Read the model definition and answer for the solid it produces. Units are mm, in the model's axes. A direction names the side the tool comes from. Coordinates: 2 decimals unless noted, no trailing zeros. Write each loop counter-clockwise with the first axis right and the second up, starting at its lowest first coordinate (ties: lowest second). Pieces come first, ordered by that corner, then holes.
Item 1: Determine the mould class of faces 1 (the face through (100, -3, 3)), 2 (the face through (1, -133.919, 3)), 3 (the face through (-76, -81, 3)) for opening direction Y: released by +Y, released by -Y, zero draft, split by the parting line, or undercut.
Item 2: Section A-A (x = 18) is taken. Give the vertices of the cut face in (y, z).
Item 3: Section B-B (y = -28) is taken. Give the vertices of the cut face in (x, z), then the cut area to 3 significant figures.
Item 4: Straight lines are drawn through the part: probe 1 along Y at (x, z) = (-11.5, 5.75); probe 2 along X at (y, z) = (-106, 5); probe 3 along X at (y, z) = (-68, 1.25). For each, find the intervals that lie inside material, in ascending order.
Item 5: Section C-C (z = 5.25) is taken. State how many separate pieces and enclosed holes the cut face has, then the cut area to 3 significant figures.
Item 6: A tool of negligible diameter and unlimited length cuts with its end or side. For faces 4 (the face through (34.308, 33.056, 3.131)), 5 (the face through (1, -29, 0)), from which of +Z, -Z, +X, -X, +Y, -Y can it reach the whole face along a straight path? Write none if from no direction.
Item 7: Each of these flat-tipped pins is pushed along its axis until it touches: P1, Ø12, axis at x = 24, y = 68, coming from the -Z side; P2, Ø3.5, axis at x = -88.37, y = -112.21, coming from the -Z side. Where does it stop, or does it pass through?
from build123d import *

# Parameters (mm, degrees)
SKETCH1_W                   = 100
SKETCH1_H                   = 265.76692074
SKETCH1_R                   = 3
BOSS_EXTRUDE2_DEPTH         = 6.35
CUTOUT_FILLETS_R            = 5
CUTOUT_FILLETS_OF_MIRROR2_R = 5


with BuildPart() as part:
    # Sketch1 → Boss-Extrude2 (new body)
    with BuildSketch(Plane.XY):
        with Locations((50, -1.035589772)):
            Rectangle(SKETCH1_W, SKETCH1_H)
        with Locations((88.366051518, 119.531107423)):
            Circle(SKETCH1_R, mode=Mode.SUBTRACT)
        with Locations((88.366051518, -0.213108197)):
            Circle(SKETCH1_R, mode=Mode.SUBTRACT)
        with Locations((88.366051518, -112.213108197)):
            Circle(SKETCH1_R, mode=Mode.SUBTRACT)
        Polygon((4, 119.786891803), (4, 71.786891803), (68, 119.786891803), align=None, mode=Mode.SUBTRACT)
        Polygon((76, 115.786891803), (12, 67.786891803), (76, 67.786891803), align=None, mode=Mode.SUBTRACT)
        Polygon((12, 59.786891803), (76, 59.786891803), (76, 11.786891803), align=None, mode=Mode.SUBTRACT)
        Polygon((68, 7.786891803), (4, 55.786891803), (4, 7.786891803), align=None, mode=Mode.SUBTRACT)
        Polygon((4, -0.213108197), (68, -0.213108197), (4, -48.213108197), align=None, mode=Mode.SUBTRACT)
        Polygon((76, -4.213108197), (12, -52.213108197), (76, -52.213108197), align=None, mode=Mode.SUBTRACT)
        Polygon((12, -60.213108197), (76, -60.213108197), (76, -108.213108197), align=None, mode=Mode.SUBTRACT)
        Polygon((4, -112.213108197), (4, -64.213108197), (68, -112.213108197), align=None, mode=Mode.SUBTRACT)
    boss_extrude2 = extrude(amount=BOSS_EXTRUDE2_DEPTH)

    # Cutout_Fillets
    cutout_fillets_edges = [part.edges().sort_by_distance(p)[0] for p in [
        (68, 119.786891803, 3.175),
        (4, 119.786891803, 3.175),
        (4, 71.786891803, 3.175),
        (76, 67.786891803, 3.175),
        (76, 115.786891803, 3.175),
        (12, 67.786891803, 3.175),
        (12, 59.786891803, 3.175),
        (76, 11.786891803, 3.175),
        (76, 59.786891803, 3.175),
        (4, 7.786891803, 3.175),
        (68, 7.786891803, 3.175),
        (4, 55.786891803, 3.175),
        (4, -0.213108197, 3.175),
        (4, -48.213108197, 3.175),
        (68, -0.213108197, 3.175),
        (76, -52.213108197, 3.175),
        (76, -4.213108197, 3.175),
        (12, -52.213108197, 3.175),
        (12, -60.213108197, 3.175),
        (76, -108.213108197, 3.175),
        (76, -60.213108197, 3.175),
        (4, -112.213108197, 3.175),
        (68, -112.213108197, 3.175),
        (4, -64.213108197, 3.175),
    ]]
    fillet(cutout_fillets_edges, radius=CUTOUT_FILLETS_R)

    # Mirror2: Boss-Extrude2 across plane
    add(boss_extrude2.mirror(Plane(origin=(0, 131.847870598, 6.35), x_dir=(0, 0, 1), z_dir=(1, 0, 0))))

    # Cutout_Fillets of Mirror2
    cutout_fillets_of_mirror2_edges = [part.edges().sort_by_distance(p)[0] for p in [
        (-68, 119.786891803, 3.175),
        (-4, 119.786891803, 3.175),
        (-4, 71.786891803, 3.175),
        (-76, 67.786891803, 3.175),
        (-76, 115.786891803, 3.175),
        (-12, 67.786891803, 3.175),
        (-12, 59.786891803, 3.175),
        (-76, 11.786891803, 3.175),
        (-76, 59.786891803, 3.175),
        (-4, 7.786891803, 3.175),
        (-68, 7.786891803, 3.175),
        (-4, 55.786891803, 3.175),
        (-4, -0.213108197, 3.175),
        (-4, -48.213108197, 3.175),
        (-68, -0.213108197, 3.175),
        (-76, -52.213108197, 3.175),
        (-76, -4.213108197, 3.175),
        (-12, -52.213108197, 3.175),
        (-12, -60.213108197, 3.175),
        (-76, -108.213108197, 3.175),
        (-76, -60.213108197, 3.175),
        (-4, -112.213108197, 3.175),
        (-68, -112.213108197, 3.175),
        (-4, -64.213108197, 3.175),
    ]]
    fillet(cutout_fillets_of_mirror2_edges, radius=CUTOUT_FILLETS_OF_MIRROR2_R)


solid = part.part
Established:
1. face 1: zero draft
1. face 2: released by -Y
1. face 3: undercut
2. outline: (-133.92, 0) - (-112.21, 0) - (-112.21, 6.35) - (-133.92, 6.35) - close; (-74.71, 0) - (-37.71, 0) - (-37.71, 6.35) - (-74.71, 6.35) - close; (-0.21, 0) - (7.79, 0) - (7.79, 6.35) - (-0.21, 6.35) - close; (45.29, 0) - (82.29, 0) - (82.29, 6.35) - (45.29, 6.35) - close; (119.79, 0) - (131.85, 0) - (131.85, 6.35) - (119.79, 6.35) - close
3. outline: (-100, 0) - (-76, 0) - (-76, 6.35) - (-100, 6.35) - close; (-44.28, 0) - (-30.95, 0) - (-30.95, 6.35) - (-44.28, 6.35) - close; (-4, 0) - (4, 0) - (4, 6.35) - (-4, 6.35) - close; (30.95, 0) - (44.28, 0) - (44.28, 6.35) - (30.95, 6.35) - close; (76, 0) - (100, 0) - (100, 6.35) - (76, 6.35) - close
3. area: 525 mm2
4. probe 1: y = -133.92 to -112.21, -69.88 to -42.54, -0.21 to 7.79, 50.12 to 77.46, 119.79 to 131.85
4. probe 2: x = -100 to -57.85, -4 to 4, 57.85 to 100
4. probe 3: x = -100 to -76, -22.85 to 22.85, 76 to 100
5. separate pieces: 1
5. enclosed holes: 22
5. area: 29,600 mm2
6. face 4: +Z, -Z
6. face 5: -Z, +X, -X, +Y, -Y
7. P1: stops at z = 0
7. P2: passes through
